```python
from build123d import *

# Parameters (mm, degrees)
SKETCH1_R           = 76.2
SKETCH1_R_2         = 50.8
SKETCH1_R_3         = 10
BOSS_EXTRUDE2_DEPTH = 25
SKETCH3_R           = 76.2
SKETCH3_R_2         = 12.7
CUT_EXTRUDE1_DEPTH  = 12.5
SKETCH4_R           = 76.2
SKETCH4_R_2         = 63.5
BOSS_EXTRUDE3_DEPTH = 15
FILLET2_R           = 2


with BuildPart() as part:
    # Sketch1 → Boss-Extrude2 (new body)
    # profile 1 of 2: a face of its own
    with BuildSketch(Plane.XY):
        Circle(SKETCH1_R)
        Circle(SKETCH1_R_2, mode=Mode.SUBTRACT)
    # profile 2 of 2: a face of its own
    with BuildSketch(Plane.XY):
        Circle(SKETCH1_R_2)
        Circle(SKETCH1_R_3, mode=Mode.SUBTRACT)
    extrude(amount=BOSS_EXTRUDE2_DEPTH)

    # Sketch3 → Cut-Extrude1 (cut, symmetric)
    with BuildSketch(Plane.XY.offset(25)):
        Circle(SKETCH3_R)
        Circle(SKETCH3_R_2, mode=Mode.SUBTRACT)
    extrude(amount=CUT_EXTRUDE1_DEPTH, both=True, mode=Mode.SUBTRACT)

    # Sketch4 → Boss-Extrude3 (add)
    with BuildSketch(Plane.XY.offset(12.5)):
        Circle(SKETCH4_R)
        Circle(SKETCH4_R_2, mode=Mode.SUBTRACT)
    extrude(amount=BOSS_EXTRUDE3_DEPTH)

    # Fillet2
    fillet2_edges = [part.edges().sort_by_distance(p)[0] for p in [
        (-76.2, 0, 27.5),
        (-76.2, 0, 0),
    ]]
    fillet(fillet2_edges, radius=FILLET2_R)


solid = part.part
```
Verification items for the finished model (mm, model axes). A direction names the side the tool comes from. Round coordinates to 2 decimals unless told otherwise and drop trailing zeros. Write each loop counter-clockwise with the first axis right and the second up, starting at its lowest first coordinate (ties: lowest second). Pieces come first, ordered by that corner, then holes. Notation, with made-up numbers: (47, 48.5) - (86, 48.5) arc R20 ccw to (86, 70.5) - close; hole circle Ø6 at (53.5, 63). An arc over 180 degrees is marked (long way). Answer as a JSON object with one key per item and string values. Group by question number.
Q1. Section check B-B, the plane z = 20.75. Enter the section's corners in (x, y), plus the area to 3 significant figures.
Q2. Section check C-C, the plane z = 10.5. Enter the section's corners in (x, y).
Q3. Mould release check, pull along Y, two halves, no side actions. Record for faces 1 (the cylindrical face through (-2.75, -12.4, 18.66)), 2 (the cylindrical face through (-60.47, -46.367, 13.586)), 3 (the cylindrical face through (-13.77, -61.99, 19.9)), 4 (the flat face through (55, 33, 27.5)): released by +Y, released by -Y, zero draft, split by the parting line, or undercut.
Q4. Tool access check on faces 5 (the flat face through (-1, -13, 12.5)), 6 (the flat face through (-1, -15, 0)). Record the directions out of +Z, -Z, +X, -X, +Y, -Y that give a thin tool (end or side, any length) a straight path to the whole face; none if there is none.
Q5. Section check A-A, the plane x = 0. Enter the section's corners in (y, z), plus the area to 3 significant figures.
Q6. Go/stop test with flat-tipped pins: pin 1 Ø12 at (x, z) = (-50.5, 7) entering from -Y; pin 2 Ø4 at (x, y) = (-31.5, 48.5) entering from +Z; pin 3 Ø1 at (y, z) = (-60.5, 18) entering from +X; pin 4 Ø2 at (x, y) = (44.5, 32) entering from -Z. Record where each tip stops, or that it passes through.
Q7. Thickness scan on line 1 (Y direction, x = 0, z = 19); line 2 (Y direction, x = 0, z = 7.5); line 3 (Z direction, x = -32.5, y = 30.5). Record the ranges inside material, lowest first.
Found:
{
 "1": {"outline": "circle Ø152.4 at (0, 0); circle Ø25.4 at (0, 0); hole circle Ø127 at (0, 0); hole circle Ø20 at (0, 0)", "area": "5,770 mm^2"},
 "2": {"outline": "circle Ø152.4 at (0, 0); hole circle Ø20 at (0, 0)"},
 "3": {"face 1": "undercut", "face 2": "split by the parting line", "face 3": "undercut", "face 4": "zero draft"},
 "4": {"face 5": "+Z", "face 6": "-Z, +X, -X, +Y, -Y"},
 "5": {"outline": "(-76.2, 2) arc R2 ccw to (-74.2, 0) - (-10, 0) - (-10, 25) - (-12.7, 25) - (-12.7, 12.5) - (-63.5, 12.5) - (-63.5, 27.5) - (-74.2, 27.5) arc R2 ccw to (-76.2, 25.5) - close; (10, 0) - (74.2, 0) arc R2 ccw to (76.2, 2) - (76.2, 25.5) arc R2 ccw to (74.2, 27.5) - (63.5, 27.5) - (63.5, 12.5) - (12.7, 12.5) - (12.7, 25) - (10, 25) - close", "area": "2,100 mm^2"},
 "6": {"pin 1": "stops at y = -61.86", "pin 2": "stops at z = 12.5", "pin 3": "stops at x = 46.97", "pin 4": "stops at z = 0"},
 "7": {"line 1": "y = -76.2 to -63.5, -12.7 to -10, 10 to 12.7, 63.5 to 76.2", "line 2": "y = -76.2 to -10, 10 to 76.2", "line 3": "z = 0 to 12.5"}
}
